from build123d import *

# Parameters (mm, degrees)
BOSS_EXTRUDE1_DEPTH  = 304.8
SHELL1_T             = -6.35
CUT_EXTRUDE1_DEPTH   = 309.49826681
RIB2_START           = -22.202989535
RIB2_DEPTH           = 44.40597907
LPATTERN1_COUNT      = 3
LPATTERN1_PITCH      = 152.4
LPATTERN2_COUNT      = 2
LPATTERN2_PITCH      = 152.4
MIRROR1_COPY_1_DEPTH = 309.49826681


# Read off the part's stored shape, not the designer's step: Rib2
with BuildPart() as part:
    # Sketch1 → Boss-Extrude1 (new, symmetric)
    with BuildSketch(Plane.XY):
        Polygon((28.575, -38.1), (-28.575, -38.1), (-25.4, 0), (25.4, 0), align=None)
    extrude(amount=BOSS_EXTRUDE1_DEPTH, both=True)

    # Shell1
    shell1_openings = [part.faces().sort_by_distance(p)[0] for p in [
        (0, -38.1, 0),
    ]]
    offset(amount=SHELL1_T, openings=shell1_openings, kind=Kind.INTERSECTION)

    # Sketch2 → Cut-Extrude1 (cut, symmetric)
    with BuildSketch(Plane(origin=(0, 0, 0), x_dir=(1, 0, 0), z_dir=(0, 1, 0))):
        with BuildLine():
            Line((4.7625, -38.1), (4.7625, -114.3))
            ThreePointArc((4.7625, -114.3), (0, -119.0625), (-4.7625, -114.3))
            Line((-4.7625, -114.3), (-4.7625, -38.1))
            ThreePointArc((-4.7625, -38.1), (0, -33.3375), (4.7625, -38.1))
        make_face()
    cut_extrude1 = extrude(amount=CUT_EXTRUDE1_DEPTH, both=True, mode=Mode.SUBTRACT)

    # Rib2 outline → Rib2 (add)
    with BuildSketch(Plane.YZ.offset(RIB2_START)):
        Polygon((-6.35, 146.447234933), (-6.35, 158.352765067), (-38.1, 155.575), (-38.1, 149.225), align=None)
    rib2 = extrude(amount=RIB2_DEPTH)

    # LPattern1: Rib2 ×3
    with Locations(*[(0, 0, -i * LPATTERN1_PITCH) for i in range(1, LPATTERN1_COUNT)]):
        add(rib2)

    # LPattern2: Cut-Extrude1 ×2
    with Locations(*[(0, 0, i * LPATTERN2_PITCH) for i in range(1, LPATTERN2_COUNT)]):
        add(cut_extrude1, mode=Mode.SUBTRACT)

    # Mirror1: Cut-Extrude1 across plane
    add(cut_extrude1.mirror(Plane.XY), mode=Mode.SUBTRACT)

    # Mirror1 copy 1 sketch → Mirror1 copy 1 (cut, symmetric)
    with BuildSketch(Plane(origin=(0, 0, -152.4), x_dir=(1, 0, 0), z_dir=(0, 1, 0))):
        with BuildLine():
            Line((4.7625, 38.1), (4.7625, 114.3))
            ThreePointArc((4.7625, 114.3), (0, 119.0625), (-4.7625, 114.3))
            Line((-4.7625, 114.3), (-4.7625, 38.1))
            ThreePointArc((-4.7625, 38.1), (0, 33.3375), (4.7625, 38.1))
        make_face()
    extrude(amount=MIRROR1_COPY_1_DEPTH, both=True, mode=Mode.SUBTRACT)


solid = part.part
CAD build for the part. Positions are in the model's coordinates, mm. A direction names the side the tool comes from. Round coordinates to 2 decimals unless told otherwise and drop trailing zeros. Write each loop counter-clockwise with the first axis right and the second up, starting at its lowest first coordinate (ties: lowest second). Pieces come first, ordered by that corner, then holes. Notation, with made-up numbers: (5.5, 89.5) -> (32.5, 89.5) arc R18 ccw to (32.5, 120.5) -> close; hole circle Ø8 at (89.5, -20.5). An arc over 180 degrees is marked (long way). Answer as a JSON object with one key per item and string values.
(1) Probe probe 1 along Z at (x, y) = (-19.5, -7); probe 2 along Z at (x, y) = (12.5, -23); probe 3 along Y at (x, z) = (2, 8.5). List the from-to ranges inside material, lowest first. Write a range as [from, to].
Reported:
{"probe 1": "z = [-304.8, -298.45], [-158.3, -146.5], [-5.9, 5.9], [146.5, 158.3], [298.45, 304.8]", "probe 2": "z = [-304.8, -298.45], [-156.9, -147.9], [-4.5, 4.5], [147.9, 156.9], [298.45, 304.8]", "probe 3": "y = [-6.35, 0]"}
(2) Band-saw the part on C-C, the plane x = -10. List the corners of the cut face in (y, z) (3 decimals).
Reported:
{"outline": "(-38.1, -304.8) -> (0, -304.8) -> (0, 304.8) -> (-38.1, 304.8) -> (-38.1, 298.45) -> (-6.35, 298.45) -> (-6.35, 158.353) -> (-38.1, 155.575) -> (-38.1, 149.225) -> (-6.35, 146.447) -> (-6.35, 5.953) -> (-38.1, 3.175) -> (-38.1, -3.175) -> (-6.35, -5.953) -> (-6.35, -146.447) -> (-38.1, -149.225) -> (-38.1, -155.575) -> (-6.35, -158.353) -> (-6.35, -298.45) -> (-38.1, -298.45) -> close"}
(3) Which spindle directions (+Z, -Z, +X, -X, +Y, -Y) get a long thin tool onto all of the face, cutting with end or side? Do faces 4 (the face through (-9, -6.35, 229)), 5 (the face through (26.965, -18.783, 4.267)). Say none if no direction does.
Reported:
{"face 4": "-Y", "face 5": "+Z, -Z, +X, +Y"}
(4) Band-saw the part on D-D, the plane z = -129.5. List the corners of the cut face in (x, y) (3 decimals), then the cut area to 3 significant figures.
Reported:
{"outline": "(-28.575, -38.1) -> (-22.203, -38.1) -> (-19.557, -6.35) -> (19.557, -6.35) -> (22.203, -38.1) -> (28.575, -38.1) -> (25.4, 0) -> (-25.4, 0) -> close", "area": "731 mm^2"}
(5) Two-plate mould, pull along Z, no slides. Class faces 1 (the face through (0, -22, 298.45)), 2 (the face through (0, -19, -304.8)), 3 (the face through (0, 0, 4)): +Z half, -Z half, draft (parallel to the pull), parting line (faces both ways), or undercut.
Reported:
{"face 1": "undercut", "face 2": "-Z half", "face 3": "draft"}
(6) Pin check, flat tips, straight feed: P1, Ø7, axis at y = -2, z = 234.5, coming from the +X side; P2, Ø1.5, axis at x = -12.5, z = -205.5, coming from the -Y side; P3, Ø7, axis at y = -4.5, z = -214, coming from the -X side. Stop position of each tip, or through.
Reported:
{"P1": "stops at x = 25.86", "P2": "stops at y = -6.35", "P3": "stops at x = -26.07"}
(7) Band-saw the part on B-B, the plane y = -22.5. List the corners of the cut face in (x, z) (3 decimals), then the cut area to 3 significant figures.
Reported:
{"outline": "(-27.275, -304.8) -> (27.275, -304.8) -> (27.275, 304.8) -> (-27.275, 304.8) -> close; hole (-20.903, -298.45) -> (20.903, -298.45) -> (20.903, -156.94) -> (-20.903, -156.94) -> close; hole (-20.903, -147.86) -> (20.903, -147.86) -> (20.903, -4.54) -> (-20.903, -4.54) -> close; hole (-20.903, 4.54) -> (20.903, 4.54) -> (20.903, 147.86) -> (-20.903, 147.86) -> close; hole (-20.903, 156.94) -> (20.903, 156.94) -> (20.903, 298.45) -> (-20.903, 298.45) -> close", "area": "9,440 mm^2"}
